Input: part model. Units: mm. Frame: model coordinates. Coordinates: 2 decimals unless noted, no trailing zeros. Write each loop counter-clockwise with the first axis right and the second up, starting at its lowest first coordinate (ties: lowest second). Pieces come first, ordered by that corner, then holes.
1) Section query C-C (z = -102). Output: boundary loops of the cut face in (x, y), then the cut area to 3 significant figures.
2) Section query A-A (y = 38.5). Output: boundary loops of the cut face in (x, z).
3) Pin query (flat end, axial travel): pin 1 Ø1.5 at (x, z) = (2, -54) entering from +Y; pin 2 Ø1.5 at (x, y) = (2, 36) entering from -Z. Return the tip coordinate at first contact, or that it passes through.
4) Section query B-B (x = 0.5). Output: boundary loops of the cut face in (y, z), then the cut area to 3 significant figures.
5) Line query: L1, parallel to Y at x = 1.6, z = -170; L2, parallel to Z at x = 1.25, y = 40; L3, parallel to Y at x = 0.8, z = -250. Output: solid intervals per line, ascending.
from build123d import *

# Parameters (mm, degrees)
SKETCH1_W           = 340
SKETCH1_H           = 20
BOSS_EXTRUDE1_DEPTH = 3
SKETCH2_R           = 2
CUT_EXTRUDE1_DEPTH  = 10
BOSS_EXTRUDE4_DEPTH = 3


with BuildPart() as part:
    # Sketch1 → Boss-Extrude1 (new body)
    with BuildSketch(Plane(origin=(0, 0, 0), x_dir=(0, 0, -1), z_dir=(1, 0, 0))):
        with Locations((170, 10)):
            Rectangle(SKETCH1_W, SKETCH1_H)
    extrude(amount=BOSS_EXTRUDE1_DEPTH)

    # Sketch2 → Cut-Extrude1 (cut)
    with BuildSketch(Plane(origin=(3, 0, 0), x_dir=(0, 0, -1), z_dir=(1, 0, 0))):
        with Locations((10, 10)):
            Circle(SKETCH2_R)
        with Locations((90, 10)):
            Circle(SKETCH2_R)
        with Locations((170, 10)):
            Circle(SKETCH2_R)
        with Locations((250, 10)):
            Circle(SKETCH2_R)
        with Locations((330, 10)):
            Circle(SKETCH2_R)
    extrude(amount=-CUT_EXTRUDE1_DEPTH, mode=Mode.SUBTRACT)

    # Sketch3 → Boss-Extrude4 (add)
    with BuildSketch(Plane(origin=(3, 0, 0), x_dir=(0, 0, -1), z_dir=(1, 0, 0))):
        with BuildLine():
            Line((160, 46), (160, 20))
            Line((160, 20), (180, 20))
            Line((180, 20), (180, 46))
            ThreePointArc((180, 46), (178.828427125, 48.828427125), (176, 50))
            Line((176, 50), (164, 50))
            ThreePointArc((164, 50), (161.171572875, 48.828427125), (160, 46))
        make_face()
        with BuildLine():
            ThreePointArc((167, 44), (170, 47), (173, 44))
            Line((173, 44), (173, 24))
            ThreePointArc((173, 24), (170, 21), (167, 24))
            Line((167, 24), (167, 44))
        make_face(mode=Mode.SUBTRACT)
    extrude(amount=-BOSS_EXTRUDE4_DEPTH)


solid = part.part
Answer:
1. outline: (0, 0) - (3, 0) - (3, 20) - (0, 20) - close
1. area: 60.0 mm2
2. outline: (0, -180) - (3, -180) - (3, -173) - (0, -173) - close; (0, -167) - (3, -167) - (3, -160) - (0, -160) - close
3. pin 1: stops at y = 20
3. pin 2: stops at z = -180
4. outline: (0, -340) - (20, -340) - (20, -180) - (46, -180) arc R4 ccw to (50, -176) - (50, -164) arc R4 ccw to (46, -160) - (20, -160) - (20, 0) - (0, 0) - close; hole circle Ø4 at (10, -330); hole circle Ø4 at (10, -250); hole circle Ø4 at (10, -170); hole circle Ø4 at (10, -90); hole circle Ø4 at (10, -10); hole (24, -173) - (44, -173) arc R3 ccw to (44, -167) - (24, -167) arc R3 ccw to start
4. area: 7,180 mm2
5. L1: y = 0 to 8, 12 to 21, 47 to 50
5. L2: z = -180 to -173, -167 to -160
5. L3: y = 0 to 8, 12 to 20
